Answer from the drawing. Dimensions are ordinates in mm from the lowest x, y and z of the part. A direction names the side the tool comes from. Coordinates: 2 decimals unless noted, no trailing zeros. Write each loop counter-clockwise with the first axis right and the second up, starting at its lowest first coordinate (ties: lowest second). Pieces come first, ordered by that corner, then holes.
1) The part is cut by section C-C (z = 19.35). Determine the outline of the cut face in (x, y).
2) Determine the mould class of the marked faces 1, 2 and 3 for opening direction X: +X half, -X half, draft (parallel to the pull), parting line (faces both ways), or undercut.
3) The part is cut by section D-D (y = 35.5). Determine the outline of the cut face in (x, z).
4) The part is cut by section A-A (y = 6.5). Determine the outline of the cut face in (x, z).
5) Which of the six approach directions +Z, -Z, +X, -X, +Y, -Y give full straight-line access (tool end or side, diameter ignored) to the marked faces 4 and 5?
6) The part is cut by section B-B (x = 19). Determine the outline of the cut face in (y, z), then the cut area to 3 significant figures.
7) Find the intervals of material crossed by line 1 (X direction, y = 34, z = 19.35); line 2 (Y direction, x = 40.5, z = 27); line 3 (Y direction, x = 36.5, z = 25.5), in increasing order.
8) Each of these flat-tipped pins is pushed along its axis until it touches: pin 1 Ø8 at (x, y) = (33, 4) entering from -Z; pin 2 Ø1.5 at (x, z) = (11.5, 27.5) entering from +Y; pin 3 Ø1.5 at (x, y) = (16.5, 18) entering from -Z (1 decimal); pin 4 Ø13 at (y, z) = (3.5, 21.5) entering from -X. Where does it stop, or does it pass through?
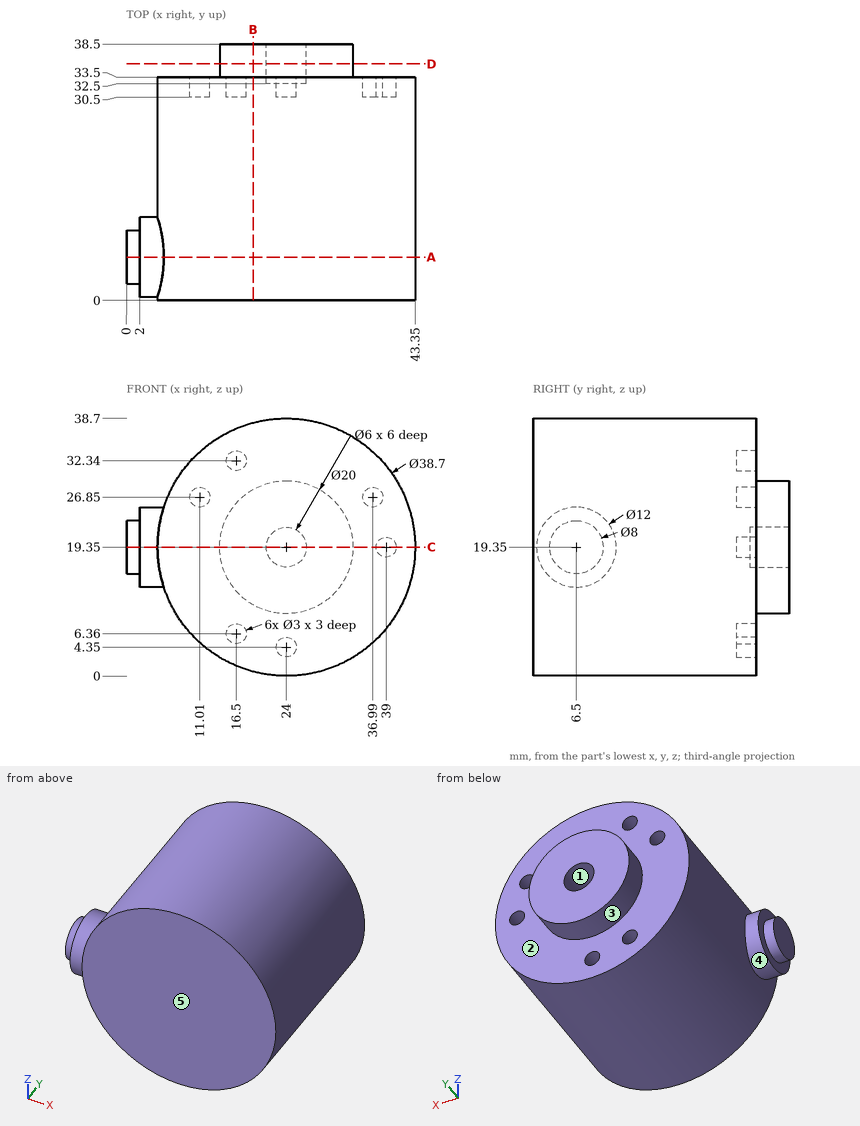
Reported:
1. outline: (0, 2.5) - (2, 2.5) - (2, 0.5) - (4.65, 0.5) - (4.65, 0) - (43.35, 0) - (43.35, 33.5) - (40.5, 33.5) - (40.5, 30.5) - (37.5, 30.5) - (37.5, 33.5) - (34, 33.5) - (34, 38.5) - (27, 38.5) - (27, 32.5) - (21, 32.5) - (21, 38.5) - (14, 38.5) - (14, 33.5) - (4.65, 33.5) - (4.65, 12.5) - (2, 12.5) - (2, 10.5) - (0, 10.5) - close
2. face 1: undercut
2. face 2: draft
2. face 3: parting line
3. outline: circle Ø20 at (24, 19.35); hole circle Ø6 at (24, 19.35)
4. outline: (0, 15.35) - (2, 15.35) - (2, 13.35) - (5.6, 13.35) arc R19.35 ccw (long way) to (5.6, 25.35) - (2, 25.35) - (2, 23.35) - (0, 23.35) - close
5. face 4: -X
5. face 5: +Z, -Z, +X, -X, -Y
6. outline: (0, 0.66) - (33.5, 0.66) - (33.5, 10.69) - (38.5, 10.69) - (38.5, 28.01) - (33.5, 28.01) - (33.5, 38.04) - (0, 38.04) - close
6. area: 1,340 mm2
7. line 1: x = 14 to 21, 27 to 34
7. line 2: y = 0 to 33.5
7. line 3: y = 0 to 30.5
8. pin 1: stops at z = 0.66
8. pin 2: stops at y = 33.5
8. pin 3: stops at z = 1.2
8. pin 4: stops at x = 0
